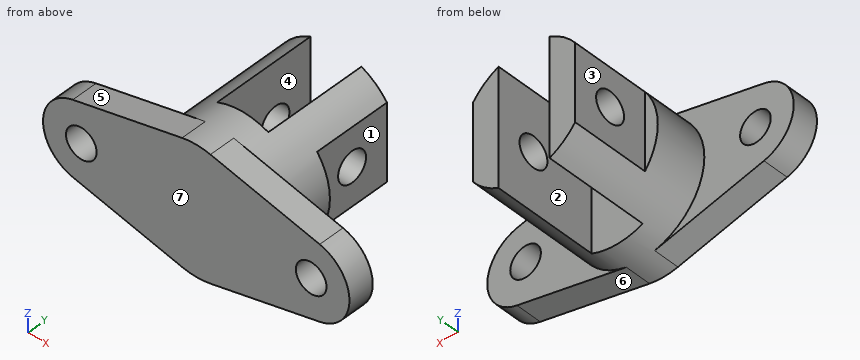
```python
from build123d import *

# Parameters (mm, degrees)
CROQUIS1_R                 = 6
SALIENTE_EXTRUIR1_DEPTH    = 10
SALIENTE_EXTRUIR1_2_DEPTH  = 10
CROQUIS1_4_R               = 25
SALIENTE_EXTRUIR2_DEPTH    = 60
CROQUIS2_W                 = 20
CROQUIS2_H                 = 56.632535906
CORTAR_EXTRUIR2_DEPTH      = 40
CROQUIS3_W                 = 5
CROQUIS3_H                 = 50
CORTAR_EXTRUIR3_DEPTH      = 30
CORTAR_EXTRUIR4_DEPTH      = 104.07764064
CORTAR_EXTRUIR4_DEPTH_BACK = 104.07764064
CROQUIS5_R                 = 6


with BuildPart() as part:
    # Croquis1 → Saliente-Extruir1 (new body)
    with BuildSketch(Plane(origin=(0, 0, 0), x_dir=(1, 0, 0), z_dir=(0, 1, 0))):
        with BuildLine():
            Line((48.333333333, 14.624940646), (5.555555556, 24.374901076))
            ThreePointArc((5.555555556, 24.374901076), (19.543398999, 15.590239112), (25, 0))
            ThreePointArc((25, 0), (19.543398999, -15.590239112), (5.555555556, -24.374901076))
            Line((5.555555556, -24.374901076), (48.333333333, -14.624940646))
            ThreePointArc((48.333333333, -14.624940646), (60, 0), (48.333333333, 14.624940646))
        make_face()
        with Locations(Location((45, 0, 0), (0, 0, 270))):
            Circle(CROQUIS1_R, mode=Mode.SUBTRACT)
    extrude(amount=SALIENTE_EXTRUIR1_DEPTH)



with BuildPart() as body_2:
    # Croquis1 → Saliente-Extruir1 2 (new body)
    with BuildSketch(Plane(origin=(0, 0, 0), x_dir=(1, 0, 0), z_dir=(0, 1, 0))):
        with BuildLine():
            Line((-5.555555556, 24.374901076), (-48.333333333, 14.624940646))
            ThreePointArc((-48.333333333, 14.624940646), (-60, 0), (-48.333333333, -14.624940646))
            Line((-48.333333333, -14.624940646), (-5.555555556, -24.374901076))
            ThreePointArc((-5.555555556, -24.374901076), (-25, 0), (-5.555555556, 24.374901076))
        make_face()
        with Locations(Location((-45, 0, 0), (0, 0, 270))):
            Circle(CROQUIS1_R, mode=Mode.SUBTRACT)
    extrude(amount=SALIENTE_EXTRUIR1_2_DEPTH)


with BuildPart() as part_1:
    add(part.part)

    add(body_2.part)  # Saliente-Extruir2 merges body 2
    # Croquis1_4 → Saliente-Extruir2 (add)
    with BuildSketch(Plane(origin=(0, 0, 0), x_dir=(1, 0, 0), z_dir=(0, 1, 0))):
        with Locations(Location((0, 0, 0), (0, 0, 77.160411593))):
            Circle(CROQUIS1_4_R)
    extrude(amount=SALIENTE_EXTRUIR2_DEPTH)

    # Croquis2 → Cortar-Extruir2 (cut)
    with BuildSketch(Plane(origin=(0, 60, 0), x_dir=(1, 0, 0), z_dir=(0, 1, 0))):
        Rectangle(CROQUIS2_W, CROQUIS2_H)
    extrude(amount=-CORTAR_EXTRUIR2_DEPTH, mode=Mode.SUBTRACT)

    # Croquis3 → Cortar-Extruir3 (cut)
    with BuildSketch(Plane(origin=(0, 60, 0), x_dir=(1, 0, 0), z_dir=(0, 1, 0))):
        with Locations((-22.5, 0)):
            Rectangle(CROQUIS3_W, CROQUIS3_H)
        with Locations((22.5, 0)):
            Rectangle(CROQUIS3_W, CROQUIS3_H)
    extrude(amount=-CORTAR_EXTRUIR3_DEPTH, mode=Mode.SUBTRACT)

    # Croquis5 → Cortar-Extruir4 (cut, two sides: drawn at the far end of the back side and taken through both)
    with BuildSketch(Plane(origin=(20, 0, 0), x_dir=(0, 0, -1), z_dir=(1, 0, 0)).offset(-CORTAR_EXTRUIR4_DEPTH_BACK)):
        with Locations((0, 45)):
            Circle(CROQUIS5_R)
    extrude(amount=CORTAR_EXTRUIR4_DEPTH + CORTAR_EXTRUIR4_DEPTH_BACK, mode=Mode.SUBTRACT)


solid = part_1.part
```
Could you check a few things on this model? Use its own coordinates, in mm. Face numbers are marked on the shaded views. A direction names the side the tool comes from. Coordinates: 2 decimals unless noted, no trailing zeros. Write each loop counter-clockwise with the first axis right and the second up, starting at its lowest first coordinate (ties: lowest second). Pieces come first, ordered by that corner, then holes. Notation, with made-up numbers: (58, 43.25) -> (76, 43.25) arc R13 cw to (76, 55.25) -> close; hole circle Ø11 at (26.5, -27.5). An arc over 180 degrees is marked (long way). Write item = value, one per line. Start each with the question number.
(1) Which directions (+Z, -Z, +X, -X, +Y, -Y) give clear straight access to the entire face, cutting with the end or side of a thin tool? Please do the marked faces 1, 2 and 3.
(2) I want a section at D-D (x = -45). Please give me the cut outline in (y, z), plus the area to 3 significant figures.
(3) We'd pull the mould along X, two halves only. Please class the marked faces 4, 5, 6 and 7: released by +X, released by -X, zero draft, split by the parting line, or undercut.
(4) I want a section at C-C (y = 45). Please give me the cut outline in (x, z).
(5) I want a section at A-A (y = 5). Please give me the cut outline in (x, z).
(6) I want a section at B-B (z = 0). Give the number of separate pieces and of enclosed holes in the cut face, plus the area to 3 significant figures.
(7) I need wall thicknesses on line 1 (X direction, y = 55.5, z = 13.5); line 2 (Y direction, x = -12.25, z = 0); line 3 (Y direction, x = -28, z = -17). Which ranges of each line are inside material? Lowest first, please. Write a range as [from, to].
(8) Will these pins go through, and if not, where does the flat tip stop? pin 1 (11 mm diameter, centred on y = 45, z = 0, fed in from -X); pin 2 (3 mm diameter, centred on x = 19.5, y = 25, fed in from +Z); pin 3 (14 mm diameter, centred on x = -45, z = 0, fed in from +Y); pin 4 (15.5 mm diameter, centred on y = 45, z = 0, fed in from +X).
Result set:
q1.face_1 = +Z, -Z, +X, +Y
q1.face_2 = +Z, -Z, +Y
q1.face_3 = +Z, -Z, -X, +Y
q2.outline = (0, -15.38) -> (10, -15.38) -> (10, -6) -> (0, -6) -> close; (0, 6) -> (10, 6) -> (10, 15.38) -> (0, 15.38) -> close
q2.area = 188 mm2
q3.face_4 = undercut
q3.face_5 = released by -X
q3.face_6 = released by +X
q3.face_7 = zero draft
q4.outline = (-20, -15) arc R25 ccw to (-10, -22.91) -> (-10, -6) -> (-20, -6) -> close; (-20, 6) -> (-10, 6) -> (-10, 22.91) arc R25 ccw to (-20, 15) -> close; (10, -22.91) arc R25 ccw to (20, -15) -> (20, -6) -> (10, -6) -> close; (10, 6) -> (20, 6) -> (20, 15) arc R25 ccw to (10, 22.91) -> close
q5.outline = (-48.33, -14.62) -> (-5.56, -24.37) arc R25 ccw to (5.56, -24.37) -> (48.33, -14.62) arc R15 ccw to (48.33, 14.62) -> (5.56, 24.37) arc R25 ccw to (-5.56, 24.37) -> (-48.33, 14.62) arc R15 ccw to start; hole circle Ø12 at (-45, 0); hole circle Ø12 at (45, 0)
q6.separate_pieces = 5
q6.enclosed_holes = 0
q6.area = 2,120 mm2
q7.line_1 = [-20, -10], [10, 20]
q7.line_2 = [0, 39], [51, 60]
q7.line_3 = [0, 10]
q8.pin_1 = through
q8.pin_2 = 17.35
q8.pin_3 = 10
q8.pin_4 = 20
